Can you work these out from the model? Positions are in its coordinate system, mm. A direction names the side the tool comes from. Round coordinates to 2 decimals unless told otherwise and drop trailing zeros. Loops run counter-clockwise (first coordinate to the right, second up) from the corner with the lowest first, then second, coordinate; pieces in that order, holes last.
```python
from build123d import *

# Parameters (mm, degrees)
F1_DEPTH = 25.4
F2_R     = 6.6675
F3_DEPTH = 12.7
F4_R     = 6.35
F5_DEPTH = 12.7


with BuildPart() as f1:
    # F0 (on Front) → F1 (new body)
    with BuildSketch(Plane.XZ):
        Polygon((-37.221345, 12.690246), (-37.719001, 0), (32.130999, 0), (32.130999, 12.690246), (13.070659, 12.690246), (13.070659, 50.790246), (-18.171345, 50.790246), (-18.171345, 12.690246), align=None)
    extrude(amount=F1_DEPTH)

    # F2 (on face) → F3 (cut)
    with BuildSketch(Plane.XY.offset(12.690246)):
        with Locations((-24.838845, -12.7)):
            Circle(F2_R)
    extrude(amount=-F3_DEPTH, mode=Mode.SUBTRACT)

    # F4 (on face) → F5 (cut)
    with BuildSketch(Plane.XY.offset(12.690246)):
        with Locations((25.609393, -14.717459)):
            Circle(F4_R)
    extrude(amount=-F5_DEPTH, mode=Mode.SUBTRACT)


solid = f1.part
```
(1) For pin 1 (9.5 mm diameter, centred on x = -32.5, y = -18, fed in from +Z); pin 2 (1 mm diameter, centred on y = -21.5, z = 43, fed in from +X); pin 3 (7.5 mm diameter, centred on y = -7.5, z = 23.5, fed in from -X), each with a flat end and sliding along its axis, tell me the tip position at first contact or that it passes through.
(2) If I drill on line 1 (Z direction, x = -22, y = -5.5); line 2 (X direction, y = -9.75, z = 19); line 3 (X direction, y = -7.5, z = 11), over which ranges is the centre line in solid material (lowest first)?
(3) Suppose I cut it at C-C (x = 14). Write out the boundary of the cut face in (y, z).
(4) Suppose I cut it at B-B (z = 16). Write out the boundary of the cut face in (x, y), then the cut area to 3 significant figures.
(5) Suppose I cut it at D-D (x = -30.5). Write out the boundary of the cut face in (y, z).
(6) Which directions (+Z, -Z, +X, -X, +Y, -Y) give clear straight access to the entire face, cutting with the end or side of a thin tool? Please do faces 1 (the flat face through (13.071, -13, 31)), 2 (the flat face through (-18.171, -13, 32)), 3 (the flat face through (-3, -25.4, 20)).
(7) We'd pull the mould along X, two halves only. Please class faces 4 (the flat face through (-32, -13, 12.69)), 5 (the cylindrical face through (-18.7, -15.3, 6.4)), 6 (the flat face through (-37.467, -12.522, 6.434)): released by +X, released by -X, zero draft, split by the parting line, or undercut.
(8) Suppose I cut it at A-A (x = 24.5). Write out the boundary of the cut face in (y, z), then the cut area to 3 significant figures.
Check result:
1. pin 1: stops at z = 12.69
1. pin 2: stops at x = 13.07
1. pin 3: stops at x = -18.17
2. line 1: z = 0 to 12.69
2. line 2: x = -18.17 to 13.07
2. line 3: x = -37.29 to -29.01, -20.67 to 32.13
3. outline: (-25.4, 0) - (0, 0) - (0, 12.69) - (-25.4, 12.69) - close
4. outline: (-18.17, -25.4) - (13.07, -25.4) - (13.07, 0) - (-18.17, 0) - close
4. area: 794 mm2
5. outline: (-25.4, 0) - (-16.22, 0) - (-16.22, 12.69) - (-25.4, 12.69) - close; (-9.18, 0) - (0, 0) - (0, 12.69) - (-9.18, 12.69) - close
6. face 1: +Z, +X, +Y, -Y
6. face 2: +Z, -X, +Y, -Y
6. face 3: +Z, -Z, +X, -X, -Y
7. face 4: zero draft
7. face 5: undercut
7. face 6: released by -X
8. outline: (-25.4, 0) - (-20.97, 0) - (-20.97, 12.69) - (-25.4, 12.69) - close; (-8.47, 0) - (0, 0) - (0, 12.69) - (-8.47, 12.69) - close
8. area: 164 mm2
